from build123d import *

# Parameters (mm, degrees)
SKETCH1_R           = 3.175
BOSS_EXTRUDE1_DEPTH = 17.526
SKETCH2_OUTSIDE_W   = 12.288
SKETCH2_OUTSIDE_H   = 12.288
SKETCH2_OUTSIDE_R   = 1.778
CUT_EXTRUDE1_DEPTH  = 10.16
SKETCH3_R           = 1.1938
CUT_EXTRUDE2_DEPTH  = 10.16
SKETCH5_R           = 0.635
CUT_EXTRUDE3_DEPTH  = 7.62
CHAMFER1_SIZE       = 0.874592138
CHAMFER1_SIZE_2     = 2.54


with BuildPart() as part:
    # Sketch1 → Boss-Extrude1 (new body)
    with BuildSketch(Plane.XY):
        Circle(SKETCH1_R)
    extrude(amount=BOSS_EXTRUDE1_DEPTH)

    # Sketch2 outside → Cut-Extrude1 (cut)
    with BuildSketch(Plane.XY.offset(17.526)):
        Rectangle(SKETCH2_OUTSIDE_W, SKETCH2_OUTSIDE_H)
        Circle(SKETCH2_OUTSIDE_R, mode=Mode.SUBTRACT)
    extrude(amount=-CUT_EXTRUDE1_DEPTH, mode=Mode.SUBTRACT)

    # Sketch3 → Cut-Extrude2 (cut)
    with BuildSketch(Plane.XY.offset(17.526)):
        Circle(SKETCH3_R)
    extrude(amount=-CUT_EXTRUDE2_DEPTH, mode=Mode.SUBTRACT)

    # Sketch5 → Cut-Extrude3 (cut)
    with BuildSketch(Plane(origin=(0, 0, 0), x_dir=(-1, 0, 0), z_dir=(0, 0, -1))):
        Circle(SKETCH5_R)
    extrude(amount=-CUT_EXTRUDE3_DEPTH, mode=Mode.SUBTRACT)

    # Chamfer1
    # the kernel refuses this chamfer: 2.54, 0.874592138 mm, written as the material it takes off along each edge
    with BuildSketch(Plane(origin=(0, 0, 0), x_dir=(1, 0, 0), z_dir=(0, -1, 0))) as chamfer1_piece_1:
        Polygon((3.175, CHAMFER1_SIZE), (3.175 - CHAMFER1_SIZE_2, 0), (3.175, 0), align=None)
    revolve(axis=Axis((0, 0, 0), (0, 0, 1)), mode=Mode.SUBTRACT)


solid = part.part
Verification items for the finished model (mm, model axes). A direction names the side the tool comes from. Give positions to 0.01 mm unless a question says otherwise; leave off trailing zeros. Write each loop counter-clockwise with the first axis right and the second up, starting at its lowest first coordinate (ties: lowest second). Pieces come first, ordered by that corner, then holes.
(1) Access from +Z, -Z, +X, -X, +Y, -Y to the whole of each face (thin tool, end or side, straight path). Record for faces 4 (the face through (0.08, 0.63, 3.63)), 5 (the face through (1, 0, 7.366)).
(2) Material ranges on line 1 (Y direction, x = 0, z = 1.5) (3 decimals); line 2 (Y direction, x = 0, z = 9.5), recorded low to high.
(3) Mould release check, pull along X, two halves, no side actions. Record for faces 1 (the face through (-0.385, -1.736, 12.517)), 2 (the face through (-0.259, -1.165, 12.517)), 3 (the face through (1.4, -1.4, 7.366)): +X half, -X half, draft (parallel to the pull), parting line (faces both ways), or undercut.
(4) Gauge pin test, flat ends, axial feed: pin 1 (2.5 mm diameter, centred on x = 0, y = -0.5, fed in from +Z); pin 2 (2 mm diameter, centred on y = -2, z = 4.5, fed in from -X); pin 3 (1.5 mm diameter, centred on y = 2, z = 11, fed in from +X). Record the tip position at first contact, or that the pin passes through.
(5) Cross-section at A-A (x = 0). Enter the section's corners in (y, z) (3 decimals).
(6) Cross-section at C-C (z = 6.25). Enter the section's corners in (x, y) (3 decimals).
Worked out:
1. face 4: +Z, -Z
1. face 5: +Z
2. line 1: y = -3.175 to -0.635, 0.635 to 3.175
2. line 2: y = -1.78 to -1.19, 1.19 to 1.78
3. face 1: parting line
3. face 2: undercut
3. face 3: draft
4. pin 1: stops at z = 17.53
4. pin 2: stops at x = -3.01
4. pin 3: stops at x = 1.26
5. outline: (-3.175, 0.875) - (-0.635, 0) - (-0.635, 7.366) - (-1.194, 7.366) - (-1.194, 17.526) - (-1.778, 17.526) - (-1.778, 7.366) - (-3.175, 7.366) - close; (0.635, 0) - (3.175, 0.875) - (3.175, 7.366) - (1.778, 7.366) - (1.778, 17.526) - (1.194, 17.526) - (1.194, 7.366) - (0.635, 7.366) - close
6. outline: circle Ø6.35 at (0, 0); hole circle Ø1.27 at (0, 0)
